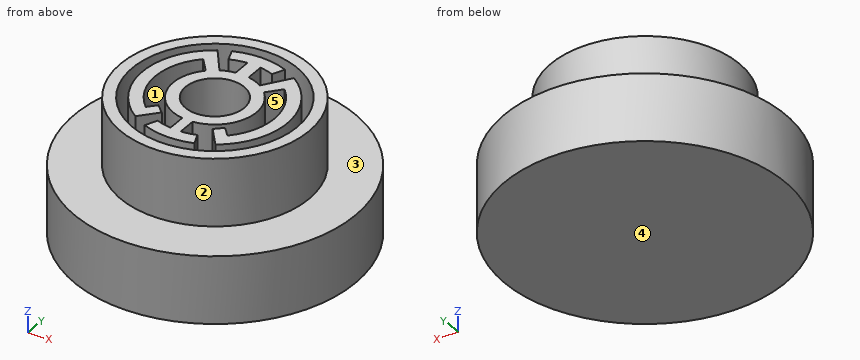
from build123d import *

# Parameters (mm, degrees)
F1_R     = 52.9315512319
F2_DEPTH = 25.4
F0_R     = 35.506963498
F0_R_2   = 31.0898313576
F0_R_3   = 11.0647908741
F3_DEPTH = 25.4


with BuildPart() as f2:
    # F1 (on Top) → F2 (new body)
    with BuildSketch(Plane.XY):
        with Locations((37.7799719572, 38.2931493223)):
            Circle(F1_R)
    extrude(amount=-F2_DEPTH)

    # F0 (on Top) → F3 (join)
    with BuildSketch(Plane.XY):
        with Locations((37.8249250984, 38.1173377679)):
            Circle(F0_R)
        with Locations((37.8249250984, 38.1173377679)):
            Circle(F0_R_2, mode=Mode.SUBTRACT)
        with BuildLine():
            Line((39.6984675691, 15.7673542773), (39.6984675691, 22.5067331888))
            ThreePointArc((39.6984675691, 22.5067331888), (52.6409755568, 32.8556093898), (49.1248120408, 49.0495695529))
            Line((49.1248120408, 49.0495695529), (53.550650699, 54.1090067787))
            ThreePointArc((53.550650699, 54.1090067787), (60.2525032987, 37.9285005747), (53.2791448176, 21.8631378094))
            Line((53.2791448176, 21.8631378094), (50.191392118, 25.1873300248))
            Line((50.191392118, 25.1873300248), (47.2831900335, 22.4859793641))
            Line((47.2831900335, 22.4859793641), (52.9763745223, 15.4227610277))
            ThreePointArc((52.9763745223, 15.4227610277), (65.1109642741, 38.4042160738), (52.4958682608, 61.1254593728))
            Line((52.4958682608, 61.1254593728), (45.8262898028, 51.651712507))
            ThreePointArc((45.8262898028, 51.651712507), (43.1781915167, 52.9005605345), (40.3444612137, 53.6367795902))
            Line((40.3444612137, 53.6367795902), (40.3444612137, 60.4037430676))
            ThreePointArc((40.3444612137, 60.4037430676), (42.9350031847, 59.9558135703), (45.4553338012, 59.2078281948))
            Line((45.4553338012, 59.2078281948), (47.4071712256, 63.6671086518))
            ThreePointArc((47.4071712256, 63.6671086518), (37.4680887103, 65.4025517281), (27.5777899968, 63.4077797425))
            Line((27.5777899968, 63.4077797425), (29.278934359, 58.8537300699))
            ThreePointArc((29.278934359, 58.8537300699), (32.2977523612, 59.8539953986), (35.4276978636, 60.4172307049))
            Line((35.4276978636, 60.4172307049), (35.4276978636, 53.6561420429))
            ThreePointArc((35.4276978636, 53.6561420429), (32.8588323546, 53.0350808805), (30.4302861837, 51.992511714))
            Line((30.4302861837, 51.992511714), (23.5229166343, 61.3565887661))
            ThreePointArc((23.5229166343, 61.3565887661), (10.5398831677, 38.487094317), (22.8984252987, 15.2741804381))
            Line((22.8984252987, 15.2741804381), (28.6635132157, 21.6562780329))
            Line((28.6635132157, 21.6562780329), (25.4403483123, 24.5678331703))
            Line((25.4403483123, 24.5678331703), (22.7109340757, 21.5463028337))
            ThreePointArc((22.7109340757, 21.5463028337), (15.3967115962, 38.0327060784), (22.5863063982, 54.5738387183))
            Line((22.5863063982, 54.5738387183), (26.9251461211, 49.4485316573))
            ThreePointArc((26.9251461211, 49.4485316573), (22.8935948893, 33.1922474233), (35.8058956554, 22.524882643))
            Line((35.8058956554, 22.524882643), (35.8058956554, 15.7800271973))
            ThreePointArc((35.8058956554, 15.7800271973), (32.9834142581, 16.2177556668), (30.2394509025, 17.0106444067))
            Line((30.2394509025, 17.0106444067), (28.214135887, 12.5782899431))
            ThreePointArc((28.214135887, 12.5782899431), (37.6196577159, 10.8305626128), (47.0504085033, 12.4365922762))
            Line((47.0504085033, 12.4365922762), (45.1568101775, 16.921220562))
            ThreePointArc((45.1568101775, 16.921220562), (42.4636561689, 16.1739082849), (39.6984675691, 15.7673542773))
        make_face()
        with Locations((37.8249250984, 38.1173377679)):
            Circle(F0_R_3, mode=Mode.SUBTRACT)
    extrude(amount=F3_DEPTH)


solid = f2.part
Work out the finished part from the listing and answer in its coordinate system (mm). Face numbers are marked on the shaded views. A direction names the side the tool comes from. Round coordinates to 2 decimals unless told otherwise and drop trailing zeros. Order: outer loops, then holes, each group sorted by start corner. A loop starts at its lowest first (then second) coordinate and runs counter-clockwise, first axis right, second up. Notation, with made-up numbers: M 81.5,3.25 L 86.5,3.25 A26 ccw 86.5,41.25 Z; hole C -15.75,48.5 d3. An arc over 180 degrees is marked long. One line per item, written item: value.
Q1. Determine the mould class of the marked faces 1, 2 and 3 for opening direction X: released by +X, released by -X, zero draft, split by the parting line, or undercut.
Derived:
face 1: undercut
face 2: split by the parting line
face 3: zero draft
Q2. Find section A-A on z = 2.5. Give the number of separate pieces and of enclosed holes in the cut face, then the cut area to 3 significant figures.
Derived:
separate pieces: 2
enclosed holes: 2
area: 2,130 mm²
Q3. Find section C-C on y = -4. Write down the section's boundary in (x, z).
Derived:
outline: M 5.95,-25.4 L 69.61,-25.4 L 69.61,0 L 5.95,0 Z
Q4. Find section D-D on z = -5. Write down the section's boundary in (x, y).
Derived:
outline: C 37.78,38.29 d105.86
Q5. Find section B-B on x = 67. Write down the section's boundary in (y, z), then the cut area to 3 significant figures.
Derived:
outline: M -5.84,-25.4 L 82.43,-25.4 L 82.43,0 L 58.35,0 L 58.35,25.4 L 48.86,25.4 L 48.86,0 L 27.38,0 L 27.38,25.4 L 17.88,25.4 L 17.88,0 L -5.84,0 Z
area: 2,720 mm²
Q6. Flat-ended cylindrical pins translate along their axes: pin 1 (5.5 mm diameter, centred on y = 17.5, z = 12, fed in from -X); pin 2 (2 mm diameter, centred on y = 56.5, z = 15, fed in from +X); pin 3 (7.5 mm diameter, centred on y = 58.5, z = 18, fed in from -X); pin 4 (12 mm diameter, centred on x = 10, y = 61, fed in from +Z). Find the tip coordinate at first contact, or state that the pin passes through.
Derived:
pin 1: x = 7.14
pin 2: x = 68.79
pin 3: x = 6.45
pin 4: z = 25.4
Q7. For the marked faces 4 and 5, determine the directions among +Z, -Z, +X, -X, +Y, -Y from which every point of the face is accessible in a straight line to the end or side of a thin tool.
Derived:
face 4: -Z, +X, -X, +Y, -Y
face 5: +Z
Q8. Straight lines are drawn through the part: line 1 (X direction, y = 38.5, z = 17); line 2 (Y direction, x = 20, z = 19.5); line 3 (Y direction, x = 58, z = 14). For each, find the intervals that lie inside material, in ascending order.
Derived:
line 1: 2.32 to 6.74, 10.54 to 15.4, 22.11 to 26.77, 48.88 to 53.54, 60.25 to 65.11, 68.91 to 73.33
line 2: 7.41 to 12.64, 17.46 to 24.5, 51.73 to 58.78, 63.59 to 68.83
line 3: 8.9 to 14.46, 19.74 to 28.32, 47.92 to 56.49, 61.77 to 67.34
